from build123d import *

# Parameters (mm, degrees)
BOSS_EXTRU_1_START      = -125
BOSS_EXTRU_1_DEPTH      = 347
ENL_V_MAT_EXTRU_1_DEPTH = 41
ENL_V_MAT_EXTRU_2_DEPTH = 41


with BuildPart() as part:
    # Esquisse1 → Boss.-Extru.1 (new body)
    with BuildSketch(Plane(origin=(0, 0, 0), x_dir=(0, 0, -1), z_dir=(1, 0, 0)).offset(BOSS_EXTRU_1_START)):
        Polygon((0, 0), (-40, 0), (-40, -17), (-17, -17), (-17, -40), (0, -40), align=None)
    extrude(amount=BOSS_EXTRU_1_DEPTH)

    # Esquisse2 → Enlèv. mat.-Extru.1 (cut, through all)
    with BuildSketch(Plane(origin=(0, 0, 0), x_dir=(1, 0, 0), z_dir=(0, 1, 0))):
        Polygon((222, 0), (182, -40), (222, -40), align=None)
    extrude(amount=-ENL_V_MAT_EXTRU_1_DEPTH, mode=Mode.SUBTRACT)

    # Esquisse3 → Enlèv. mat.-Extru.2 (cut, through all)
    with BuildSketch(Plane(origin=(0, 0, 0), x_dir=(-1, 0, 0), z_dir=(0, 0, -1))):
        Polygon((-222, 0), (-182, -40), (-222, -40), align=None)
    extrude(amount=-ENL_V_MAT_EXTRU_2_DEPTH, mode=Mode.SUBTRACT)


solid = part.part
Read the model definition and answer for the solid it produces. Units are mm, in the model's axes. A direction names the side the tool comes from. Round coordinates to 2 decimals unless told otherwise and drop trailing zeros. Order: outer loops, then holes, each group sorted by start corner. A loop starts at its lowest first (then second) coordinate and runs counter-clockwise, first axis right, second up. Notation, with made-up numbers: (-13.75, -6.75) - (44.25, -6.75) arc R16 cw to (44.25, 15.25) - close; hole circle Ø9 at (-32.75, 78.5). An arc over 180 degrees is marked (long way). Use one line per item in the form item = value. Start each with the question number.
(1) The part is cut by section B-B (z = 8). Give the vertices of the cut face in (x, y), then the cut area to 3 significant figures.
(2) The part is cut by section A-A (y = -3). Give the vertices of the cut face in (x, z), then the cut area to 3 significant figures.
(3) Find the intervals of material crossed by line 1 along Z through (x, y) = (122, -26); line 2 along Y through (x, z) = (-82, 19); line 3 along X through (y, z) = (-16, 27), in increasing order. Write a range as from..to.
(4) The part is cut by section D-D (y = -28.5). Give the vertices of the cut face in (x, z).
(5) Flat-ended cylindrical pins translate along their axes: pin 1 Ø12 at (y, z) = (-25.5, 29) entering from -X; pin 2 Ø6 at (y, z) = (-20, 7) entering from +X; pin 3 Ø11.5 at (x, y) = (31.5, -27) entering from +Z; pin 4 Ø3 at (x, z) = (74.5, 34) entering from -Y. Find the tip coordinate at first contact, or state that the pin passes through.
(6) The part is cut by section C-C (x = 157). Give the vertices of the cut face in (y, z).
(7) For faces 1 (the face through (38, -17, 29)), 2 (the face through (198, -24, 8)), determine the directions among +Z, -Z, +X, -X, +Y, -Y from which every point of the face is accessible in a straight line to the end or side of a thin tool.
Checked values:
q1.outline = (-125, -40) - (182, -40) - (214, -8) - (214, 0) - (-125, 0) - close
q1.area = 13,000 mm^2
q2.outline = (-125, 0) - (219, 0) - (219, 3) - (182, 40) - (-125, 40) - close
q2.area = 13,100 mm^2
q3.line_1 = 0..17
q3.line_2 = -17..0
q3.line_3 = -125..195
q4.outline = (-125, 0) - (193.5, 0) - (193.5, 17) - (-125, 17) - close
q5.pin_1 = through
q5.pin_2 = 205
q5.pin_3 = 17
q5.pin_4 = -17
q6.outline = (-40, 0) - (0, 0) - (0, 40) - (-17, 40) - (-17, 17) - (-40, 17) - close
q7.face_1 = +Z, +X, -X, -Y
q7.face_2 = +Z, -Z, +X, -Y
